Geometry check sheet. Reference: the model listing, model coordinates, mm. Give positions to 0.01 mm unless a question says otherwise; leave off trailing zeros. Write each loop counter-clockwise with the first axis right and the second up, starting at its lowest first coordinate (ties: lowest second). Pieces come first, ordered by that corner, then holes. Notation, with made-up numbers: (-8.75, 12) -> (6.25, 12) arc R11 cw to (6.25, 20) -> close; hole circle Ø7 at (14.25, 75.5). An arc over 180 degrees is marked (long way). One line per item, written item: value.
from build123d import *

# Parameters (mm, degrees)
SKETCH1_R           = 2
SKETCH1_R_2         = 1.5
BOSS_EXTRUDE1_DEPTH = 5
SKETCH3_R           = 4.5
CUT_EXTRUDE1_DEPTH  = 3.5
SKETCH7_R           = 1
CUT_EXTRUDE3_DEPTH  = 10
SKETCH10_R          = 1.499999992
CUT_EXTRUDE4_DEPTH  = 108.72827842


with BuildPart() as part:
    # Sketch1 → Boss-Extrude1 (new body)
    with BuildSketch(Plane.XY):
        with BuildLine():
            Line((8.662544735, 63.892298354), (8.662544735, 8.892298354))
            Line((8.662544735, 8.892298354), (-6.337455265, 8.892298354))
            Line((-6.337455265, 8.892298354), (-6.337455265, 68.892298354))
            Line((-6.337455265, 68.892298354), (1.556032109, 99.524396458))
            ThreePointArc((1.556032109, 99.524396458), (15.487791899, 104.147761306), (15.253774048, 89.470749723))
            Line((15.253774048, 89.470749723), (8.662544735, 63.892298354))
        make_face()
        with Locations((10.162544735, 96.892298354)):
            Circle(SKETCH1_R, mode=Mode.SUBTRACT)
        with Locations((1.162544735, 43.892298354)):
            Circle(SKETCH1_R_2, mode=Mode.SUBTRACT)
    extrude(amount=BOSS_EXTRUDE1_DEPTH)

    # Sketch3 → Cut-Extrude1 (cut)
    with BuildSketch(Plane(origin=(0, 0, 0), x_dir=(-1, 0, 0), z_dir=(0, 0, -1))):
        with Locations((-10.162544735, 96.892298354)):
            Circle(SKETCH3_R)
    extrude(amount=-CUT_EXTRUDE1_DEPTH, mode=Mode.SUBTRACT)

    # Sketch7 → Cut-Extrude3 (cut)
    with BuildSketch(Plane(origin=(0, 0, 0), x_dir=(-1, 0, 0), z_dir=(0, 0, -1))):
        with Locations((-3.063597883, 70.045794856)):
            Circle(SKETCH7_R)
        with Locations((1.794946815, 74.363727627)):
            Circle(SKETCH7_R)
    extrude(amount=-CUT_EXTRUDE3_DEPTH, mode=Mode.SUBTRACT)

    # Sketch10 → Cut-Extrude4 (cut, through all)
    with BuildSketch(Plane(origin=(0, 0, 0), x_dir=(-1, 0, 0), z_dir=(0, 0, -1))):
        with Locations((2.337455106, 59.512300154)):
            Circle(SKETCH10_R)
        with Locations((-4.662544922, 59.512300154)):
            Circle(SKETCH10_R)
    extrude(amount=-CUT_EXTRUDE4_DEPTH, mode=Mode.SUBTRACT)


solid = part.part
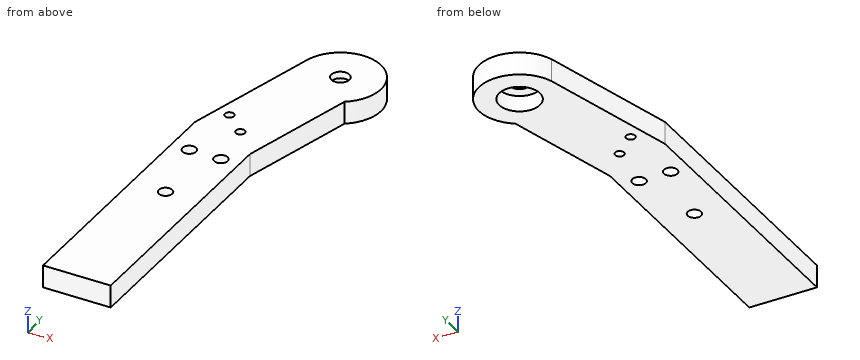
1) Sectioned sample at B-B on x = 13.75. Record the cut outline in (y, z).
Verdict:
outline: (83.64, 0) -> (94.18, 0) -> (94.18, 3.5) -> (99.61, 3.5) -> (99.61, 0) -> (105.15, 0) -> (105.15, 5) -> (83.64, 5) -> close
2) Sectioned sample at C-C on y = 35. Record the cut outline in (x, z), plus the area to 3 significant figures.
Verdict:
outline: (-6.34, 0) -> (8.66, 0) -> (8.66, 5) -> (-6.34, 5) -> close
area: 75.0 mm^2
3) Depth check by flat-ended pin: pin 1 Ø2.5 at (y, z) = (31, 2) entering from +X; pin 2 Ø1.5 at (x, y) = (7.5, 49) entering from -Z; pin 3 Ø3 at (x, y) = (10.16, 96.89) entering from -Z; pin 4 Ø2 at (y, z) = (78.5, 3.5) entering from -X. Enter the tip coordinate at first touch or a pass-through.
Verdict:
pin 1: x = 8.66
pin 2: z = 0
pin 3: through
pin 4: x = -4.12
4) Sectioned sample at A-A on z = 2.55. Record the cut outline in (x, y).
Verdict:
outline: (-6.34, 8.89) -> (8.66, 8.89) -> (8.66, 63.89) -> (15.25, 89.47) arc R9 ccw (long way) to (1.56, 99.52) -> (-6.34, 68.89) -> close; hole circle Ø3 at (-2.34, 59.51); hole circle Ø2 at (-1.79, 74.36); hole circle Ø3 at (1.16, 43.89); hole circle Ø2 at (3.06, 70.05); hole circle Ø3 at (4.66, 59.51); hole circle Ø9 at (10.16, 96.89)
5) Scan lines: probe 1 along Y at (x, z) = (2.25, 1.7); probe 2 along Y at (x, z) = (3.75, 0.3); probe 3 along X at (y, z) = (58.5, 1.45). Record each from-to range of solid material in increasing order.
Verdict:
probe 1: 8.89 to 42.86, 44.93 to 69.46, 70.63 to 101.18
probe 2: 8.89 to 58.32, 60.7 to 69.32, 70.77 to 103.21
probe 3: -6.34 to -3.44, -1.23 to 3.56, 5.77 to 8.66
6) Sectioned sample at D-D on y = 88.5. Record the cut outline in (x, z), plus the area to 3 significant figures.
Verdict:
outline: (-1.28, 0) -> (15, 0) -> (15, 5) -> (-1.28, 5) -> close
area: 81.4 mm^2
